from build123d import *

# Parameters (mm, degrees)
SKETCH5_W           = 185
SKETCH5_H           = 185
BOSS_EXTRUDE5_DEPTH = 30
SKETCH6_W           = 55
SKETCH6_H           = 55
CUT_EXTRUDE2_DEPTH  = 10
SKETCH7_R           = 20
CUT_EXTRUDE3_DEPTH  = 167.353137545
SKETCH8_W           = 175
SKETCH8_H           = 175
CUT_EXTRUDE4_DEPTH  = 15
SKETCH9_W           = 165
SKETCH9_H           = 15
CUT_EXTRUDE6_DEPTH  = 225.262725022
SKETCH11_W          = 15
SKETCH11_H          = 165
CUT_EXTRUDE7_DEPTH  = 218.323713701


with BuildPart() as part:
    # Sketch5 → Boss-Extrude5 (new body)
    with BuildSketch(Plane.XY):
        with Locations((30.661559889, 17.520891365)):
            Rectangle(SKETCH5_W, SKETCH5_H)
    extrude(amount=BOSS_EXTRUDE5_DEPTH)

    # Sketch6 → Cut-Extrude2 (cut)
    with BuildSketch(Plane(origin=(0, 0, 0), x_dir=(-1, 0, 0), z_dir=(0, 0, -1))):
        with Locations((29.338440111, 17.520891365)):
            Rectangle(SKETCH6_W, SKETCH6_H)
        with Locations((29.338440111, -42.479108635)):
            Rectangle(SKETCH6_W, SKETCH6_H)
        with Locations((-30.661559889, -42.479108635)):
            Rectangle(SKETCH6_W, SKETCH6_H)
        with Locations((-30.661559889, 17.520891365)):
            Rectangle(SKETCH6_W, SKETCH6_H)
        with Locations((-30.661559889, 77.520891365)):
            Rectangle(SKETCH6_W, SKETCH6_H)
        with Locations((-90.661559889, 77.520891365)):
            Rectangle(SKETCH6_W, SKETCH6_H)
        with Locations((-90.661559889, 17.520891365)):
            Rectangle(SKETCH6_W, SKETCH6_H)
        with Locations((-90.661559889, -42.479108635)):
            Rectangle(SKETCH6_W, SKETCH6_H)
        with Locations((29.338440111, 77.520891365)):
            Rectangle(SKETCH6_W, SKETCH6_H)
    extrude(amount=-CUT_EXTRUDE2_DEPTH, mode=Mode.SUBTRACT)

    # Sketch7 → Cut-Extrude3 (cut, through all)
    with BuildSketch(Plane(origin=(0, 0, 10), x_dir=(-1, 0, 0), z_dir=(0, 0, -1))):
        with Locations((-90.661559889, 77.520891365)):
            Circle(SKETCH7_R)
        with Locations((-30.661559889, 77.520891365)):
            Circle(SKETCH7_R)
        with Locations((29.338440111, 77.520891365)):
            Circle(SKETCH7_R)
        with Locations((29.338440111, 17.520891365)):
            Circle(SKETCH7_R)
        with Locations((-30.661559889, 17.520891365)):
            Circle(SKETCH7_R)
        with Locations((-90.661559889, 17.520891365)):
            Circle(SKETCH7_R)
        with Locations((29.338440111, -42.479108635)):
            Circle(SKETCH7_R)
        with Locations((-90.661559889, -42.479108635)):
            Circle(SKETCH7_R)
        with Locations((-30.661559889, -42.479108635)):
            Circle(SKETCH7_R)
    extrude(amount=-CUT_EXTRUDE3_DEPTH, mode=Mode.SUBTRACT)

    # Sketch8 → Cut-Extrude4 (cut)
    with BuildSketch(Plane.XY.offset(30)):
        with Locations((30.661559889, 17.520891365)):
            Rectangle(SKETCH8_W, SKETCH8_H)
    extrude(amount=-CUT_EXTRUDE4_DEPTH, mode=Mode.SUBTRACT)

    # Sketch9 → Cut-Extrude6 (cut, through all)
    with BuildSketch(Plane(origin=(0, 110.020891365, 0), x_dir=(1, 0, 0), z_dir=(0, 1, 0))):
        with Locations((30.661559889, -22.5)):
            Rectangle(SKETCH9_W, SKETCH9_H)
    extrude(amount=-CUT_EXTRUDE6_DEPTH, mode=Mode.SUBTRACT)

    # Sketch11 → Cut-Extrude7 (cut, through all)
    with BuildSketch(Plane.ZY.offset(61.838440111)):
        with Locations((22.5, 17.520891365)):
            Rectangle(SKETCH11_W, SKETCH11_H)
    extrude(amount=-CUT_EXTRUDE7_DEPTH, mode=Mode.SUBTRACT)


solid = part.part
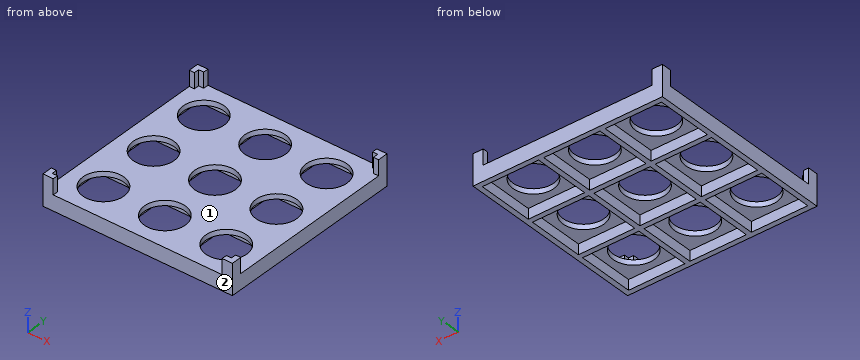
Design review of the part built by this model. Coordinates are the model's own, in mm. Face numbers are marked on the shaded views. Coordinates: 2 decimals unless noted, no trailing zeros. Order: outer loops, then holes, each group sorted by start corner. A loop starts at its lowest first (then second) coordinate and runs counter-clockwise, first axis right, second up.
Item 1: Take a section at A-A, the plane z = 18.25. Write out the cut boundary in (x, y).
Item 2: Take a section at C-C, the plane y = -39.5. Write out the cut boundary in (x, z), then the cut area to 3 significant figures.
Item 3: For line 1 (Y direction, x = -32, z = 5.5); line 2 (X direction, y = -30, z = 5); line 3 (Y direction, x = 31.5, z = 13.75), list the stretches that pass through material, from the lowest coordinate up.
Item 4: The part is to be moulded in two halves that separate along X. For the marked faces 1 and 2, say which applies: pulls with the +X half, pulls with the -X half, needs draft (parallel to the pull), parting line crosses it, or undercut.
Item 5: Take a section at B-B, the plane x = 19. Write out the cut boundary in (y, z), then the cut area to 3 significant figures.
Item 6: For pin 1 Ø4 at (x, y) = (101, -26.5) entering from +Z, flat-tipped, find the tip position at first contact; note if it passes through.
Item 7: Take a section at D-D, the plane x = 55.5. Write out the cut boundary in (y, z).
The answers:
1. outline: (-61.84, -74.98) - (-51.84, -74.98) - (-51.84, -69.98) - (-56.84, -69.98) - (-56.84, -64.98) - (-61.84, -64.98) - close; (-61.84, 100.02) - (-56.84, 100.02) - (-56.84, 105.02) - (-51.84, 105.02) - (-51.84, 110.02) - (-61.84, 110.02) - close; (113.16, -74.98) - (123.16, -74.98) - (123.16, -64.98) - (118.16, -64.98) - (118.16, -69.98) - (113.16, -69.98) - close; (113.16, 105.02) - (118.16, 105.02) - (118.16, 100.02) - (123.16, 100.02) - (123.16, 110.02) - (113.16, 110.02) - close
2. outline: (-61.84, 0) - (-56.84, 0) - (-56.84, 10) - (-49.12, 10) - (-49.12, 15) - (-61.84, 15) - close; (-9.56, 10) - (-1.84, 10) - (-1.84, 0) - (3.16, 0) - (3.16, 10) - (10.88, 10) - (10.88, 15) - (-9.56, 15) - close; (50.44, 10) - (58.16, 10) - (58.16, 0) - (63.16, 0) - (63.16, 10) - (70.88, 10) - (70.88, 15) - (50.44, 15) - close; (110.44, 10) - (118.16, 10) - (118.16, 0) - (123.16, 0) - (123.16, 15) - (110.44, 15) - close
2. area: 532 mm2
3. line 1: y = -74.98 to -69.98, -14.98 to -9.98, 45.02 to 50.02, 105.02 to 110.02
3. line 2: x = -61.84 to -56.84, -1.84 to 3.16, 58.16 to 63.16, 118.16 to 123.16
3. line 3: y = -74.98 to -62.46, -22.5 to -2.46, 37.5 to 57.54, 97.5 to 110.02
4. face 1: undercut
4. face 2: needs draft
5. outline: (-74.98, 0) - (-69.98, 0) - (-69.98, 10) - (-58.73, 10) - (-58.73, 15) - (-74.98, 15) - close; (-26.23, 10) - (-14.98, 10) - (-14.98, 0) - (-9.98, 0) - (-9.98, 10) - (1.27, 10) - (1.27, 15) - (-26.23, 15) - close; (33.77, 10) - (45.02, 10) - (45.02, 0) - (50.02, 0) - (50.02, 10) - (61.27, 10) - (61.27, 15) - (33.77, 15) - close; (93.77, 10) - (105.02, 10) - (105.02, 0) - (110.02, 0) - (110.02, 15) - (93.77, 15) - close
5. area: 638 mm2
6. pin 1: stops at z = 15
7. outline: (-74.98, 0) - (-69.98, 0) - (-69.98, 10) - (-14.98, 10) - (-14.98, 0) - (-9.98, 0) - (-9.98, 10) - (45.02, 10) - (45.02, 0) - (50.02, 0) - (50.02, 10) - (105.02, 10) - (105.02, 0) - (110.02, 0) - (110.02, 15) - (-74.98, 15) - close
